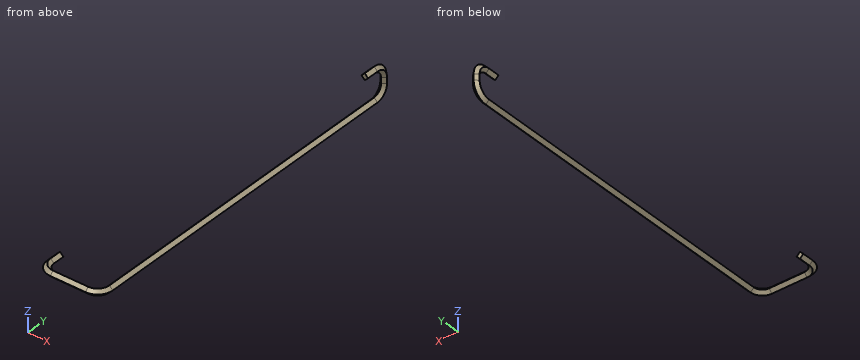
from build123d import *


with BuildPart() as f4:
    # F4: sweep along a path in F0, F2
    with BuildLine(Plane.XY) as f4_path:
        Line((0, 0), (0, -20))
        ThreePointArc((0, -20), (5.8578643763, -34.1421356237), (20, -40))
        Line((20, -40), (80, -40))
        ThreePointArc((80, -40), (94.1421356237, -34.1421356237), (100, -20))
        Line((100, -20), (100, 540))
    with BuildLine(Plane.YZ.offset(100)) as f4_path_2:
        ThreePointArc((540, 0), (554.1421356237, 5.8578643763), (560, 20))
        Line((560, 20), (560, 30))
        ThreePointArc((560, 30), (554.1421356237, 44.1421356237), (540, 50))
        Line((540, 50), (520, 50))
    # F3 (on Front) → F4 (sweep)
    with BuildSketch(Plane.XZ):
        Polygon((0, -5.6568542495), (5.6568542495, 0), (0, 5.6568542495), (-5.6568542495, 0), align=None)
    sweep(path=f4_path.line + f4_path_2.line)


solid = f4.part
Work out the finished part from the listing and answer in its coordinate system (mm). Coordinates: 2 decimals unless noted, no trailing zeros. Loops run counter-clockwise (first coordinate to the right, second up) from the corner with the lowest first, then second, coordinate; pieces in that order, holes last. Notation, with made-up numbers: M -10,35.25 L 29,35.25 A16 ccw 29,57.25 Z; hole C 13.25,48.25 d1. An arc over 180 degrees is marked long. Answer in a Markdown table with one row per item. Add a question column.
1. Find section A-A, the plane x = 50. Write down the section's boundary in (y, z), then the cut area to 3 significant figures.
2. Consider L1, parallel to X at y = 75.5, z = 5.5; L2, parallel to X at y = 531, z = 53.5; L3, parallel to Z at x = 100.5, y = 323.5. Determine where each line is inside the solid, lowest interval first.
3. Flat-ended cylindrical pins translate along their axes: P1, Ø12.5, axis at x = 98, z = 49, coming from the -Y side; P2, Ø10, axis at x = 14, z = 4.5, coming from the -Y side; P3, Ø1, axis at x = 93, y = 189.5, coming from the -Z side; P4, Ø10, axis at x = 79, z = 10, coming from the +Y side. Find the tip coordinate at first contact, or state that the pin passes through.
4. Find section B-B, the plane y = 226. Write down the section's boundary in (x, z), then the cut area to 3 significant figures.
Reported:
| question | item | result |
|---|---|---|
| 1 | outline | M -45.66,0 L -40,-5.66 L -34.34,0 L -40,5.66 Z |
| 1 | area | 64.0 mm^2 |
| 2 | L1 | x = 99.84 to 100.16 |
| 2 | L2 | x = 97.84 to 102.16 |
| 2 | L3 | z = -5.16 to 5.16 |
| 3 | P1 | stops at y = 520 |
| 3 | P2 | stops at y = -45.37 |
| 3 | P3 | passes through |
| 3 | P4 | stops at y = -39.34 |
| 4 | outline | M 94.34,0 L 100,-5.66 L 105.66,0 L 100,5.66 Z |
| 4 | area | 64.0 mm^2 |
